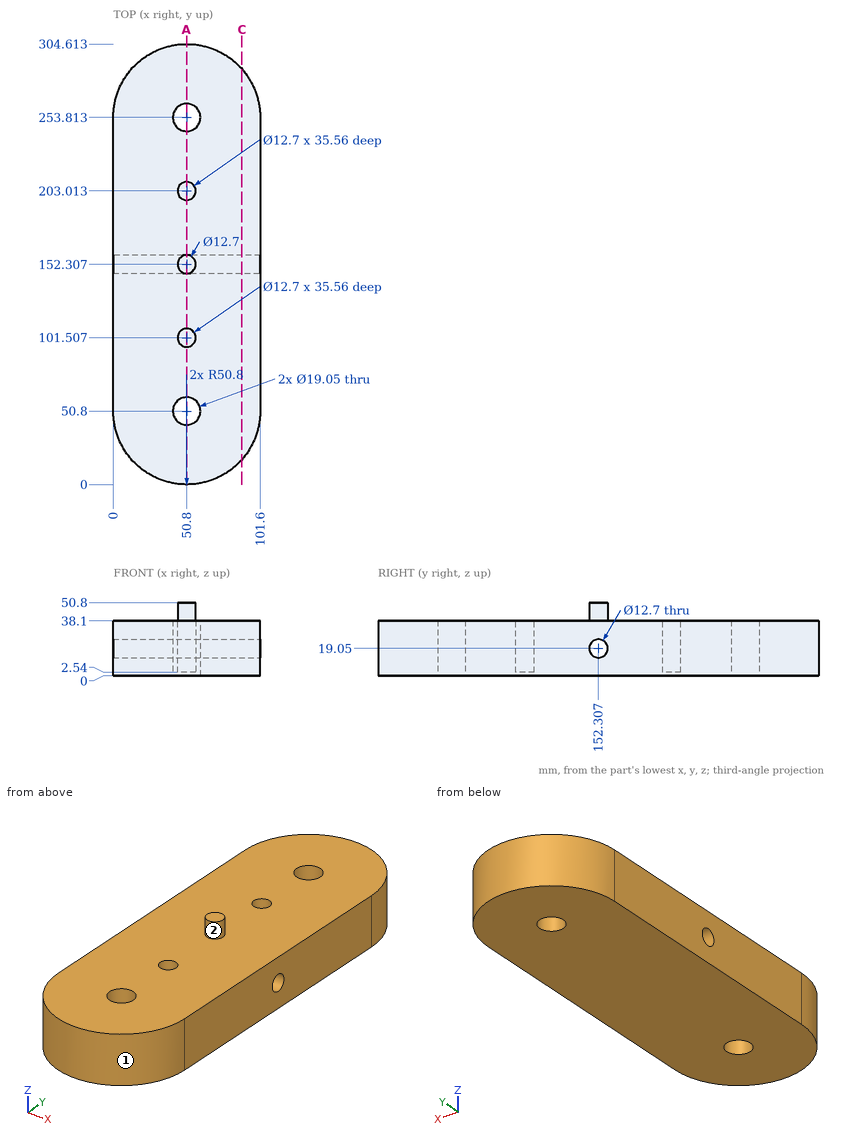
Geometry: see drawing. Coordinates: mm, zero at the bounding-box minimum. A direction names the side the tool comes from. Round coordinates to 2 decimals unless told otherwise and drop trailing zeros. Loops run counter-clockwise (first coordinate to the right, second up) from the corner with the lowest first, then second, coordinate; pieces in that order, holes last. Notation, with made-up numbers: (-11, -7.5) -> (27, -7.5) arc R22 cw to (27, 17.5) -> close; hole circle Ø11 at (85.5, 66). An arc over 180 degrees is marked (long way). Write each question's results on one line, items separated by ' | '.
1. Set-up query: the marked faces 1 and 2. Return all of +Z, -Z, +X, -X, +Y, -Y with unobstructed straight access to the full face (end or side cutting, diameter ignored); none if empty.
Geometry results:
face 1: +Z, -Z, -Y | face 2: +Z
2. Section C-C (x = 89). Return loops of the section in (y, z).
Geometry results:
outline: (17.31, 0) -> (287.3, 0) -> (287.3, 38.1) -> (17.31, 38.1) -> close; hole circle Ø12.7 at (152.31, 19.05)
3. First-contact query: P1, Ø11.5, axis at x = 50.8, y = 50.8, coming from the -Z side; P2, Ø12, axis at x = 48, z = 34.5, coming from the +Y side; P3, Ø14, axis at x = 50, y = 99, coming from the +Z side; P4, Ø10, axis at x = 50.8, y = 101.51, coming from the +Z side. Flat tips, straight axial feed; report the tip coordinate or a pass-through.
Geometry results:
P1: through | P2: y = 304.61 | P3: z = 38.1 | P4: z = 2.54
4. Ray query, line 1 (X direction, y = 203.5, z = 16.5); line 2 (Y direction, x = 50.8, z = 12.5) (1 decimal); line 3 (Z direction, x = 65.5, y = 125). Return the intervals inside material, ascending. Write a range as from..to.
Geometry results:
line 1: 0..44.47, 57.13..101.6 | line 2: 0..41.3, 60.3..95.2, 107.9..196.7, 209.4..244.3, 263.3..304.6 | line 3: 0..38.1
5. Section A-A (x = 50.8). State how many separate pieces and enclosed holes the cut face has.
Geometry results:
separate pieces: 3 | enclosed holes: 1
